The model under review builds one solid part; all positions refer to its coordinate system, in mm. Face numbers are marked on the shaded views. A direction names the side the tool comes from. Coordinates: 2 decimals unless noted, no trailing zeros. Write each loop counter-clockwise with the first axis right and the second up, starting at its lowest first coordinate (ties: lowest second). Pieces come first, ordered by that corner, then holes. Notation, with made-up numbers: (70, -12) -> (81, -12) arc R28 cw to (81, 13) -> close; hole circle Ø4 at (14, 69.25). An arc over 180 degrees is marked (long way). Put each result on its own line as item: value. Start each with the question number.
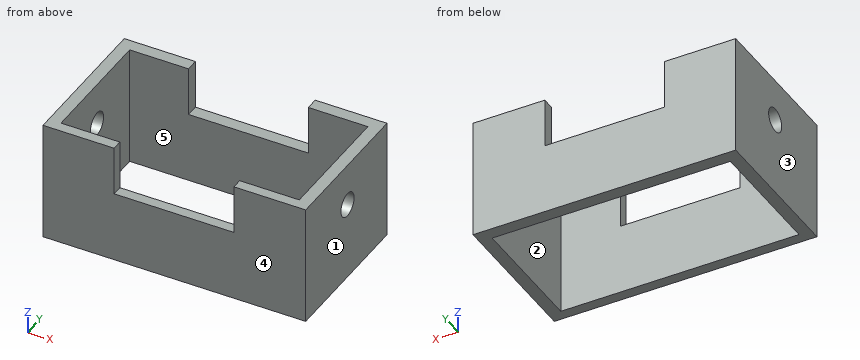
from build123d import *

# Parameters (mm, degrees)
F0_W      = 276.7956107855
F0_H      = 155.8074429631
F1_DEPTH  = 127
F2_R      = 12.5546361004
F3_DEPTH  = 276.7966107855
F4_W      = 126.266527921
F4_H      = 51.968123436
F5_DEPTH  = 155.8084429631
F6_W      = 251.0117739439
F6_H      = 131.5910294652
F7_DEPTH  = 75.032876564
F8_W      = 61.992302537
F8_H      = 58.8230818466
F9_DEPTH  = 51.969123436
F10_W     = 61.992302537
F10_H     = 52.2348090963
F11_DEPTH = 51.969123436
F12_W     = 62.752943486
F12_H     = 58.8230818466
F13_DEPTH = 51.969123436
F14_W     = 62.752943486
F14_H     = 52.2348090963
F15_DEPTH = 51.969123436
F16_W     = 61.992302537
F16_H     = 20.5331385223
F17_DEPTH = 127.001
F18_W     = 62.752943486
F18_H     = 20.5331385223
F19_DEPTH = 127.001


with BuildPart() as f1:
    # F0 (on Top) → F1 (new body)
    with BuildSketch(Plane.XY):
        with Locations((-4.9713328481, -2.2223033011)):
            Rectangle(F0_W, F0_H)
    extrude(amount=F1_DEPTH)

    # F2 (on face) → F3 (cut, through all)
    with BuildSketch(Plane.YZ.offset(133.4264725447)):
        with Locations((0, 82.2579711676)):
            Circle(F2_R)
    extrude(amount=-F3_DEPTH, mode=Mode.SUBTRACT)

    # F4 (on face) → F5 (cut, through all)
    with BuildSketch(Plane(origin=(0, 75.6814181805, 0), x_dir=(-1, 0, 0), z_dir=(0, 1, 0))):
        with Locations((5.3516533226, 101.015938282)):
            Rectangle(F4_W, F4_H)
    extrude(amount=-F5_DEPTH, mode=Mode.SUBTRACT)

    # F6 (on face) → F7 (cut, through all)
    with BuildSketch(Plane.XY.offset(75.031876564)):
        with Locations((-4.9713328481, -3.2941363752)):
            Rectangle(F6_W, F6_H)
    extrude(amount=-F7_DEPTH, mode=Mode.SUBTRACT)

    # F8 (on face) → F9 (cut, through all)
    with BuildSketch(Plane(origin=(0, 0, 75.031876564), x_dir=(1, 0, 0), z_dir=(0, 0, -1))):
        with Locations((-99.4810685515, 39.6781101845)):
            Rectangle(F8_W, F8_H)
    extrude(amount=-F9_DEPTH, mode=Mode.SUBTRACT)

    # F10 (on face) → F11 (cut, through all)
    with BuildSketch(Plane(origin=(0, 0, 75.031876564), x_dir=(1, 0, 0), z_dir=(0, 0, -1))):
        with Locations((-99.4810685515, -36.3839738093)):
            Rectangle(F10_W, F10_H)
    extrude(amount=-F11_DEPTH, mode=Mode.SUBTRACT)

    # F12 (on face) → F13 (cut, through all)
    with BuildSketch(Plane(origin=(0, 0, 75.031876564), x_dir=(1, 0, 0), z_dir=(0, 0, -1))):
        with Locations((89.1580823809, 39.6781101845)):
            Rectangle(F12_W, F12_H)
    extrude(amount=-F13_DEPTH, mode=Mode.SUBTRACT)

    # F14 (on face) → F15 (cut, through all)
    with BuildSketch(Plane(origin=(0, 0, 75.031876564), x_dir=(1, 0, 0), z_dir=(0, 0, -1))):
        with Locations((89.1580823809, -36.3839738093)):
            Rectangle(F14_W, F14_H)
    extrude(amount=-F15_DEPTH, mode=Mode.SUBTRACT)

    # F16 (on face) → F17 (cut, through all)
    with BuildSketch(Plane.XY.offset(127)):
        with Locations((-99.4810685515, 0)):
            Rectangle(F16_W, F16_H)
    extrude(amount=-F17_DEPTH, mode=Mode.SUBTRACT)

    # F18 (on face) → F19 (cut, through all)
    with BuildSketch(Plane.XY.offset(127)):
        with Locations((89.1580823809, 0)):
            Rectangle(F18_W, F18_H)
    extrude(amount=-F19_DEPTH, mode=Mode.SUBTRACT)


solid = f1.part
1. Consider section D-D on y = -17.5. State the section outline as (x, z) points, then the cut area to 3 significant figures.
2. Wall thickness on line 1 (Y direction, x = -92.5, z = 94); line 2 (Z direction, x = -139.25, y = 0); line 3 (X direction, y = -32, z = 31.5): over which ranges is each line inside the solid? List them lowest first. Write a range as from..to.
3. Tool access review of the marked faces 1 and 2: name each direction out of +Z, -Z, +X, -X, +Y, -Y from which nothing blocks a thin tool from reaching the whole face with its end or side.
4. Consider section C-C on z = 34. State the section outline as (x, y) points, then the cut area to 3 significant figures.
5. Insertion check: P1, Ø9, axis at x = 26, y = -74.5, coming from the +Z side. The pin has a flat end and moves straight along its axis. Give the tip position at first contact, or say it passes through.
6. Consider section B-B on y = 0. State the section outline as (x, z) points.
7. The part is to be moulded in two halves that separate along X. For the marked faces 3, 4 and 5, say which applies: released by +X, released by -X, zero draft, split by the parting line, or undercut.
8. Consider section A-A on x = 79.5. State the section outline as (y, z) points.
Output values:
1. outline: (-143.37, 0) -> (-130.48, 0) -> (-130.48, 127) -> (-143.37, 127) -> close; (120.53, 0) -> (133.43, 0) -> (133.43, 127) -> (120.53, 127) -> close
1. area: 3,270 mm^2
2. line 1: y = -80.13..-69.09, 62.5..75.68
2. line 2: z = 0..69.7, 94.81..127
2. line 3: x = -143.37..-130.48, 120.53..133.43
3. face 1: +Z, -Z, +X, +Y, -Y
3. face 2: +Z, -Z
4. outline: (-143.37, -80.13) -> (133.43, -80.13) -> (133.43, 75.68) -> (-143.37, 75.68) -> close; hole (-130.48, -69.09) -> (120.53, -69.09) -> (120.53, 62.5) -> (-130.48, 62.5) -> close
4. area: 10,100 mm^2
5. P1: stops at z = 75.03
6. outline: (-143.37, 0) -> (-130.48, 0) -> (-130.48, 69.7) -> (-143.37, 69.7) -> close; (-143.37, 94.81) -> (-130.48, 94.81) -> (-130.48, 127) -> (-143.37, 127) -> close; (120.53, 0) -> (133.43, 0) -> (133.43, 69.7) -> (120.53, 69.7) -> close; (120.53, 94.81) -> (133.43, 94.81) -> (133.43, 127) -> (120.53, 127) -> close
7. face 3: released by -X
7. face 4: zero draft
7. face 5: undercut
8. outline: (-80.13, 0) -> (-69.09, 0) -> (-69.09, 127) -> (-80.13, 127) -> close; (62.5, 0) -> (75.68, 0) -> (75.68, 127) -> (62.5, 127) -> close
